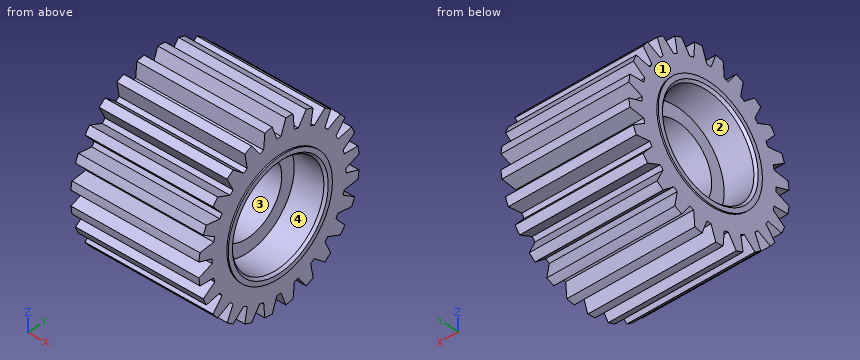
```python
from build123d import *

# Parameters (mm, degrees)
SCHNITT_LINEAR_AUSTRAGEN1_REACH = 41.29
KREISMUSTER1_COUNT              = 24


with BuildPart() as part:
    # Skizze1 → Rotation1 (revolve)
    with BuildSketch(Plane.XY, mode=Mode.PRIVATE) as rotation1_sk:
        Polygon((-14.3, 12.5), (-14.3, 11.5), (-13.8, 11), (-7.3, 11), (-7.3, 8), (7.3, 8), (7.3, 11), (13.8, 11), (14.3, 11.5), (14.3, 12.5), (14, 12.5), (14, 19.2715), (-14, 19.2715), (-14, 12.5), align=None)
    revolve(rotation1_sk.sketch.rotate(Axis((-36.010442658, 0, 0), (1, 0, 0)), 90), axis=Axis((-36.010442658, 0, 0), (1, 0, 0)))

    # Skizze2 → Schnitt-Linear austragen1 (cut, up to next)
    with BuildSketch(Plane(origin=(14, 0, 0), x_dir=(0, 0, -1), z_dir=(1, 0, 0)), mode=Mode.PRIVATE) as schnitt_linear_austragen1_sk1:
        with BuildLine():
            Line((0.491939129, 16.076475108), (1.629707388, 19.202467708))
            ThreePointArc((1.629707388, 19.202467708), (0, 19.2715), (-1.629707388, 19.202467708))
            Line((-1.629707388, 19.202467708), (-0.491939129, 16.076475108))
            ThreePointArc((-0.491939129, 16.076475108), (0, 16.084), (0.491939129, 16.076475108))
        make_face()
    schnitt_linear_austragen1_tool1 = extrude(schnitt_linear_austragen1_sk1.sketch, amount=-SCHNITT_LINEAR_AUSTRAGEN1_REACH, mode=Mode.PRIVATE) & part.part
    schnitt_linear_austragen1 = schnitt_linear_austragen1_tool1.solids().sort_by_distance((14, 17.949237, 0))[0]
    add(schnitt_linear_austragen1, mode=Mode.SUBTRACT)

    # Kreismuster1: Schnitt-Linear austragen1 ×24 about axis
    kreismuster1_axis = Axis((0, 0, 0), (1, 0, 0))
    for i in range(1, KREISMUSTER1_COUNT):
        add(schnitt_linear_austragen1.rotate(kreismuster1_axis, i * 360 / KREISMUSTER1_COUNT), mode=Mode.SUBTRACT)


solid = part.part
```
Here's how the part is built. I have some questions about the finished solid (model axes, mm). Face numbers are marked on the shaded views. A direction names the side the tool comes from. Give positions to 0.01 mm unless a question says otherwise; leave off trailing zeros. Write each loop counter-clockwise with the first axis right and the second up, starting at its lowest first coordinate (ties: lowest second). Pieces come first, ordered by that corner, then holes. Notation, with made-up numbers: M 24,87 L 43,87 A17 ccw 43,99 Z; hole C 52,49 d9. An arc over 180 degrees is marked long. Put each result on its own line as item: value. Start each with the question number.
Item 1: If we section it at C-C, the plane z = 13: Write out the boundary of the cut face in (x, y), then the cut area to 3 significant figures.
Item 2: If we section it at A-A, the plane y = 0: Write out the boundary of the cut face in (x, z), then the cut area to 3 significant figures.
Item 3: Will these pins go through, and if not, where does the flat tip stop? pin 1 (4 mm diameter, centred on y = 8, z = -3.5, fed in from +X); pin 2 (6.5 mm diameter, centred on y = 5, z = 0, fed in from -X); pin 3 (10 mm diameter, centred on x = 0.5, y = 3.5, fed in from -Z).
Item 4: I need wall thicknesses on L1, parallel to Y at x = -6.75, z = 15; L2, parallel to Y at x = 0.25, z = 0; L3, parallel to Y at x = -11.75, z = 0. Which ranges of each line are inside material? Lowest first, please. Write a range as from..to.
Item 5: On a 3-axis mill with a long thin cutter (end or side, diameter ignored), from which of +Z, -Z, +X, -X, +Y, -Y can I reach the whole of each face in a straight line? I mean the marked faces 3 and 4. Say none if no direction works.
Item 6: Thinking about a two-plate mould opening in Z: for the marked faces 1 and 2, which applies, +Z half, -Z half, draft (parallel to the pull), parting line (faces both ways), or undercut?
Values:
1. outline: M -14,-11.62 L 14,-11.62 L 14,11.62 L -14,11.62 Z
1. area: 651 mm²
2. outline: M -14.3,-12.5 L -14,-12.5 L -14,-16.08 L 14,-16.08 L 14,-12.5 L 14.3,-12.5 L 14.3,-11.5 L 13.8,-11 L 7.3,-11 L 7.3,-8 L -7.3,-8 L -7.3,-11 L -13.8,-11 L -14.3,-11.5 Z; M -14.3,11.5 L -13.8,11 L -7.3,11 L -7.3,8 L 7.3,8 L 7.3,11 L 13.8,11 L 14.3,11.5 L 14.3,12.5 L 14,12.5 L 14,16.08 L -14,16.08 L -14,12.5 L -14.3,12.5 Z
2. area: 374 mm²
3. pin 1: x = 7.3
3. pin 2: x = -7.3
3. pin 3: z = -19.2
4. L1: -12.1..-10.04, -7.76..7.76, 10.04..12.1
4. L2: -16.08..-8, 8..16.08
4. L3: -16.08..-11, 11..16.08
5. face 3: +X, -X
5. face 4: +X
6. face 1: draft
6. face 2: undercut
